The model under review builds one solid part; all positions refer to its coordinate system, in mm. A direction names the side the tool comes from. Give positions to 0.01 mm unless a question says otherwise; leave off trailing zeros. Loops run counter-clockwise (first coordinate to the right, second up) from the corner with the lowest first, then second, coordinate; pieces in that order, holes last. Notation, with made-up numbers: M -20.5,10 L 14.5,10 A24 cw 14.5,27 Z; hole C 83,10 d2. An arc over 180 degrees is marked long. Return JSON: item names as keys, results as strings.
```python
from build123d import *

# Parameters (mm, degrees)
SKETCH2_W                                      = 5
SKETCH2_H                                      = 60
EXTRUDE_THIN1_DEPTH                            = 60
SKETCH3_R                                      = 5
SKETCH4_R                                      = 3.5
CUT_EXTRUDE1_DEPTH                             = 137.839321834
CSK_FOR_M8_FLAT_HEAD_MACHINE_SCREW1_AT_2_COUNT = 2
CSK_FOR_M8_FLAT_HEAD_MACHINE_SCREW1_AT_2_PITCH = 27.483528756


with BuildPart() as part:
    # Sketch2 → Extrude-Thin1 (new, symmetric)
    with BuildSketch(Plane.XY):
        with Locations((2.5, 30)):
            Rectangle(SKETCH2_W, SKETCH2_H)
    extrude(amount=EXTRUDE_THIN1_DEPTH, both=True)

    # Sweep11: sweep along a curve in space
    with BuildLine() as sweep11_path:
        Line((5, 60, 60), (5, 60, -60))
    # Sketch3 → Sweep11 (sweep)
    with BuildSketch(Plane.XY.offset(60)):
        with Locations((5, 60)):
            Circle(SKETCH3_R)
    sweep(path=sweep11_path.line)

    # Sketch4 → Cut-Extrude1 (cut, through all)
    with BuildSketch(Plane.XY.offset(60)):
        with Locations((5, 60)):
            Circle(SKETCH4_R)
    extrude(amount=-CUT_EXTRUDE1_DEPTH, mode=Mode.SUBTRACT)

    # Sketch6 → CSK for M8 Flat Head Machine Screw1 (revolve, cut)
    with BuildSketch(Plane(origin=(5, 35.505970187, 44.516987054), x_dir=(0, 0, -1), z_dir=(0, 1, 0))):
        Polygon((0, 0), (0, 5), (4.5, 5), (4.5, 5.15), (8.65, 1), (8.65, 0), align=None)
    csk_for_m8_flat_head_machine_screw1 = revolve(axis=Axis((11.35, 35.505970187, 44.516987054), (-1, 0, 0)), mode=Mode.SUBTRACT)

    # CSK for M8 Flat Head Machine Screw1 at 2: CSK for M8 Flat Head Machine Screw1 ×2
    with Locations(*[Vector(0, -0.7968641919109715, -0.604158472298514) * (i * CSK_FOR_M8_FLAT_HEAD_MACHINE_SCREW1_AT_2_PITCH) for i in range(1, CSK_FOR_M8_FLAT_HEAD_MACHINE_SCREW1_AT_2_COUNT)]):
        add(csk_for_m8_flat_head_machine_screw1, mode=Mode.SUBTRACT)

    # Mirror1: CSK for M8 Flat Head Machine Screw1 across plane
    add(csk_for_m8_flat_head_machine_screw1.mirror(Plane.XY), mode=Mode.SUBTRACT)

    # Mirror1 copy 1 sketch → Mirror1 copy 1 (revolve, cut)
    with BuildSketch(Plane(origin=(5, 13.605330254, -27.912580307), x_dir=(0, 0, 1), z_dir=(0, 1, 0))):
        Polygon((0, 0), (0, -5), (4.5, -5), (4.5, -5.15), (8.65, -1), (8.65, 0), align=None)
    revolve(axis=Axis((11.35, 13.605330254, -27.912580307), (1, 0, 0)), mode=Mode.SUBTRACT)


solid = part.part
```
1) Consider section C-C on y = 24. Write out the cut boundary in (x, z), then the cut area to 3 significant figures.
From the geometry:
{"outline": "M 0,-60 L 5,-60 L 5,60 L 0,60 Z", "area": "600 mm²"}
2) Consider section B-B on z = 26.5. Count the separate pieces of the cut face and the enclosed holes in it, then the cut area to 3 significant figures.
From the geometry:
{"separate pieces": "2", "enclosed holes": "1", "area": "251 mm²"}
3) Consider section A-A on x = 2.75. Write out the cut boundary in (y, z), then the cut area to 3 significant figures.
From the geometry:
{"outline": "M 0,-60 L 57.32,-60 L 57.32,60 L 0,60 Z; M 62.68,-60 L 64.47,-60 L 64.47,60 L 62.68,60 Z; hole C 13.61,-27.91 d14.8; hole C 13.61,27.91 d14.8; hole C 35.51,-44.52 d14.8; hole C 35.51,44.52 d14.8", "area": "6,400 mm²"}
4) Tool access review of faces 1 (the face through (5, 27, 1)), 2 (the face through (4.507, 13.225, -36.554)), 3 (the face through (8, 64, -1)): name each direction out of +Z, -Z, +X, -X, +Y, -Y from which nothing blocks a thin tool from reaching the whole face with its end or side.
From the geometry:
{"face 1": "+Z, -Z, +X, -Y", "face 2": "+X", "face 3": "+Z, -Z"}
5) The part is to be moulded in two halves that separate along Z. For faces 4 (the face through (4.51, 11.01, 19.66)), 5 (the face through (0, 30, 1)), 6 (the face through (3, 33, 60)), say which applies: released by +Z, released by -Z, zero draft, split by the parting line, or undercut.
From the geometry:
{"face 4": "undercut", "face 5": "zero draft", "face 6": "released by +Z"}
6) Insertion check: pin 1 (15.5 mm diameter, centred on y = 13.61, z = -27.91, fed in from +X); pin 2 (10 mm diameter, centred on y = 44.5, z = -27.5, fed in from +X). Each pin has a flat end and moves straight along its axis. Give the tip position at first contact, or say it passes through.
From the geometry:
{"pin 1": "x = 3.11", "pin 2": "x = 5"}
7) Wall thickness on L1, parallel to Y at x = 3.5, z = 27; L2, parallel to Y at x = 3.5, z = -43.5; L3, parallel to X at y = 20.5, z = 13: over which ranges is each line inside the solid? List them lowest first. Write a range as from..to.
From the geometry:
{"L1": "0..5.51, 21.7..56.84, 63.16..64.77", "L2": "0..27.42, 43.59..56.84, 63.16..64.77", "L3": "0..5"}
